Design review of the part built by this model. Coordinates are the model's own, in mm. Coordinates: 2 decimals unless noted, no trailing zeros. Loops run counter-clockwise (first coordinate to the right, second up) from the corner with the lowest first, then second, coordinate; pieces in that order, holes last. Notation, with made-up numbers: M -40,-15.5 L -19,-15.5 A12 cw -19,4.5 Z; hole C 27.5,51.5 d8. An arc over 180 degrees is marked long. Put each result on its own line as item: value. Start each with the question number.
(1) Clearance check with flat-ended pins moving along their axes: pin 1 (1.8 mm diameter, centred on x = 168, z = 3.5, fed in from -Y); pin 2 (1.8 mm diameter, centred on x = -37.5, z = 3.5, fed in from +Y); pin 3 (3 mm diameter, centred on y = 62, z = 3, fed in from -X). State where each tip first meets the part, or that it passes through.
(2) For probe 1 along Y at (x, z) = (111, 0.8); probe 2 along X at (y, z) = (11, 3.4), list the stretches that pass through material, from the lowest coordinate up. Write a range as [from, to].
(3) Take a section at A-A, the plane y = 15. Give the boundary of the cut face in (x, z), then the cut area to 3 significant figures.
Autodesk Inventor part; units mm, degrees
ref_plane "YZ Plane" through (0, 0, 0) normal (1, 0, 0) x (0, 1, 0)
ref_plane "XZ Plane" through (0, 0, 0) normal (0, 1, 0) x (-1, 0, 0)
ref_plane "XY Plane" through (0, 0, 0) normal (0, 0, 1) x (1, 0, 0)
ref_plane "Work Plane1" through (0, 0, 0) normal (0, 0, 1) x (1, 0, 0)
sketch "Sketch1" plane through (0, 0, 0) normal (0, 0, 1) x (1, 0, 0)
  line L0 (-34, 6) -> (-34, 0)
  line L1 (-34, 0) -> (0, 0)
  line L2 (0, 0) -> (0, 6)
  line L3 (0, 6) -> (-34, 6)
  line L4 (0, 6) -> (30, 6)
  line L5 (0, 0) -> (0, 6)
  line L6 (30, 0) -> (0, 0)
  line L7 (30, 0) -> (30, 6)
  line L8 (30, 6) -> (30, 0)
  line L9 (30, 0) -> (60, 0)
  line L10 (60, 0) -> (60, 6)
  line L11 (60, 6) -> (30, 6)
  line L12 (60, 6) -> (90, 6)
  line L13 (60, 0) -> (60, 6)
  line L14 (90, 0) -> (60, 0)
  line L15 (90, 0) -> (90, 6)
  line L16 (90, 6) -> (90, 0)
  line L17 (90, 0) -> (120, 0)
  line L18 (120, 0) -> (120, 6)
  line L19 (120, 6) -> (90, 6)
  line L20 (120, 6) -> (150, 6)
  line L21 (120, 0) -> (120, 6)
  line L22 (150, 0) -> (120, 0)
  line L23 (150, 0) -> (150, 6)
  line L24 (150, 6) -> (150, 0)
  line L25 (150, 0) -> (180, 0)
  line L26 (180, 0) -> (180, 6)
  line L27 (180, 6) -> (150, 6)
  line L28 (180, 6) -> (210, 6)
  line L29 (180, 6) -> (210, 6)
  line L30 (180, 0) -> (180, 6)
  line L31 (210, 0) -> (180, 0)
  line L32 (210, 0) -> (210, 6)
  line L33 (240, 0) -> (240, 6)
  line L34 (240, 6) -> (210, 6)
  line L35 (210, 6) -> (210, 0)
  line L36 (210, 0) -> (240, 0)
  line L37 (240, 6) -> (270, 6)
  line L38 (240, 0) -> (240, 6)
  line L39 (270, 0) -> (240, 0)
  line L40 (270, 0) -> (270, 6)
  line L41 (300, 0) -> (300, 6)
  line L42 (300, 6) -> (270, 6)
  line L43 (270, 6) -> (270, 0)
  line L44 (270, 0) -> (300, 0)
  line L45 (300, 6) -> (330, 6)
  line L46 (300, 0) -> (300, 6)
  line L47 (330, 0) -> (300, 0)
  line L48 (330, 0) -> (330, 6)
  line L49 (360, 0) -> (360, 6)
  line L50 (360, 6) -> (330, 6)
  line L51 (330, 6) -> (330, 0)
  line L52 (330, 0) -> (360, 0)
  line L53 (360, 6) -> (390, 6)
  line L54 (360, 0) -> (360, 6)
  line L55 (390, 0) -> (360, 0)
  line L56 (390, 0) -> (390, 6)
  line L57 (424, 0) -> (424, 6)
  line L58 (424, 6) -> (390, 6)
  line L59 (390, 6) -> (390, 0)
  line L60 (390, 0) -> (424, 0)
  line L61 (-34, 6) -> (424, 6)
  line L62 (424, 6) -> (424, 76)
  line L63 (424, 76) -> (-34, 76)
  line L64 (-34, 76) -> (-34, 6)
  line L65 (401, 57.7) -> (300, 57.7)
  line L66 (-34, 53.5) -> (-40, 53.5)
  line L67 (-40, 53.5) -> (-40, 28.5)
  line L68 (-40, 28.5) -> (-34, 28.5)
  line L69 (-34, 28.5) -> (-34, 53.5)
  line L70 (424, 53.5) -> (430, 53.5)
  line L71 (430, 53.5) -> (430, 28.5)
  line L72 (430, 28.5) -> (424, 28.5)
  line L73 (424, 28.5) -> (424, 53.5)
  point P0 (430, 41)
  point P1 (424, 41)
  point P2 (-40, 41)
  point P3 (-34, 41)
  point P4 (-34, 41)
  dimension "d0" = 70
  dimension "d2" = 6
  dimension "d3" = 6
  dimension "d4" = 25
extrude "Plate1" add sketch "Sketch1" along normal blind 6 contours L64 L63 L62 L58 L53 L50 L45 L42 L37 L34 L28 L27 L20 L19 L12 L11 L4 L3 | L4 L7 L6 L2 | L68 L67 L66 L64 | L12 L15 L14 L10 | L20 L23 L22 L18 | L70 L71 L72 L62 | L28 L32 L31 L26 | L56 L55 L49 L53 | L37 L40 L39 L33 | L48 L47 L41 L45
equation "\"d1\" = Thickness"
equation "\"BendRadius\" = Thickness"
equation "\"BendReliefWidth\" = Thickness"
equation "\"BendReliefDepth\" = 0.5 * Thickness"
equation "\"CornerReliefSize\" = 4 * Thickness"
equation "\"MinimumRemnant\" = 2 * Thickness"
equation "\"TransitionRadius\" = BendRadius"
equation "\"JacobiRadiusSize\" = BendRadius"
equation "\"GapSize\" = Thickness"
properties part number "voorzijde boven elektrobox v2" material "Wood (Birch)"
Computed values:
1. pin 1: stops at y = 6
1. pin 2: stops at y = 53.5
1. pin 3: stops at x = -34
2. probe 1: y = [6, 76]
2. probe 2: x = [-34, 424]
3. outline: M -34,0 L 424,0 L 424,6 L -34,6 Z
3. area: 2,750 mm^2
